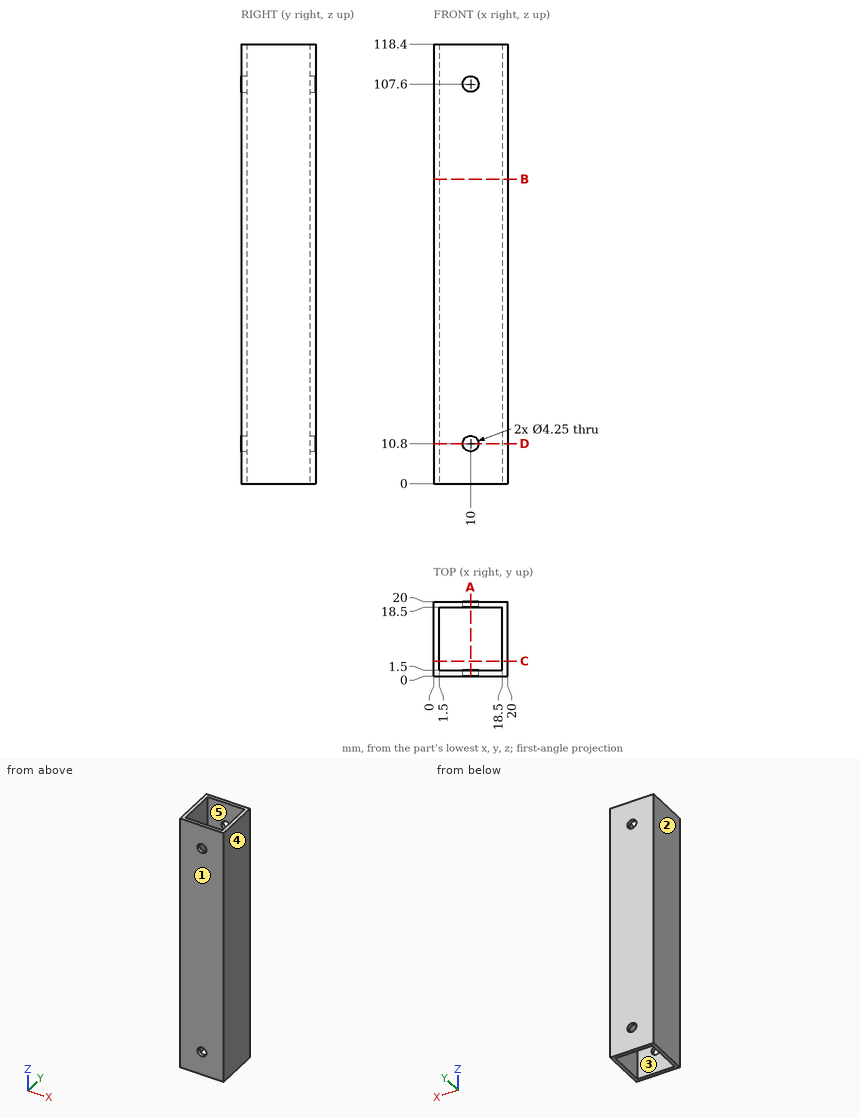
Design review of the part shown in the three views and the two pictorial views. Dimensions are in mm from the part's minimum x, y and z. A direction names the side the tool comes from. Round coordinates to 2 decimals unless told otherwise and drop trailing zeros. Write each loop counter-clockwise with the first axis right and the second up, starting at its lowest first coordinate (ties: lowest second). Pieces come first, ordered by that corner, then holes. Notation, with made-up numbers: (37.5, 72) -> (49.5, 72) arc R19 cw to (49.5, 99) -> close; hole circle Ø6 at (65, 63.25). An arc over 180 degrees is marked (long way). Answer as a JSON object with one key per item and string values.
1. Machinability: for the marked faces 4 and 5, which of the approach directions +Z, -Z, +X, -X, +Y, -Y give a long, thin tool a straight path to every point of the face, cutting with its end or side? Answer none if there is none.
Results found:
{"face 4": "+Z, -Z, +X, +Y, -Y", "face 5": "+Z, -Z"}
2. We need section A-A on x = 10. State the section outline as (y, z) points (3 decimals).
Results found:
{"outline": "(0, 0) -> (1.5, 0) -> (1.5, 8.675) -> (0, 8.675) -> close; (0, 12.925) -> (1.5, 12.925) -> (1.5, 105.475) -> (0, 105.475) -> close; (0, 109.725) -> (1.5, 109.725) -> (1.5, 118.4) -> (0, 118.4) -> close; (18.5, 0) -> (20, 0) -> (20, 8.675) -> (18.5, 8.675) -> close; (18.5, 12.925) -> (20, 12.925) -> (20, 105.475) -> (18.5, 105.475) -> close; (18.5, 109.725) -> (20, 109.725) -> (20, 118.4) -> (18.5, 118.4) -> close"}
3. To check wall thickness, follow line 1 along X through (y, z) = (15.5, 70.5); line 2 along X through (y, z) = (0.3, 10.8) (3 decimals). State the ranges of each line that lie inside material, in increasing order.
Results found:
{"line 1": "x = 0 to 1.5, 18.5 to 20", "line 2": "x = 0 to 7.875, 12.125 to 20"}
4. We need section B-B on z = 82. State the section outline as (x, y) points.
Results found:
{"outline": "(0, 0) -> (20, 0) -> (20, 20) -> (0, 20) -> close; hole (1.5, 1.5) -> (18.5, 1.5) -> (18.5, 18.5) -> (1.5, 18.5) -> close"}
5. We need section D-D on z = 10.8. State the section outline as (x, y) points (3 decimals), and give its area (4 significant figures).
Results found:
{"outline": "(0, 0) -> (7.875, 0) -> (7.875, 1.5) -> (1.5, 1.5) -> (1.5, 18.5) -> (7.875, 18.5) -> (7.875, 20) -> (0, 20) -> close; (12.125, 0) -> (20, 0) -> (20, 20) -> (12.125, 20) -> (12.125, 18.5) -> (18.5, 18.5) -> (18.5, 1.5) -> (12.125, 1.5) -> close", "area": "98.25 mm^2"}
6. The part is to be moulded in two halves that separate along X. For the marked faces 1, 2 and 3, say which applies: pulls with the +X half, pulls with the -X half, needs draft (parallel to the pull), parting line crosses it, or undercut.
Results found:
{"face 1": "needs draft", "face 2": "pulls with the -X half", "face 3": "undercut"}
7. We need section C-C on y = 4. State the section outline as (x, z) points, and give its area (3 significant figures).
Results found:
{"outline": "(0, 0) -> (1.5, 0) -> (1.5, 118.4) -> (0, 118.4) -> close; (18.5, 0) -> (20, 0) -> (20, 118.4) -> (18.5, 118.4) -> close", "area": "355 mm^2"}
